Design review of the part built by this model. Coordinates are the model's own, in mm. Face numbers are marked on the shaded views. Give positions to 0.01 mm unless a question says otherwise; leave off trailing zeros. Loops run counter-clockwise (first coordinate to the right, second up) from the corner with the lowest first, then second, coordinate; pieces in that order, holes last. Notation, with made-up numbers: (85, 56.25) - (118, 56.25) arc R22 ccw to (118, 93.25) - close; hole circle Ø2 at (-9.75, -33.5). An arc over 180 degrees is marked (long way). Write each question's results on one line, items separated by ' | '.
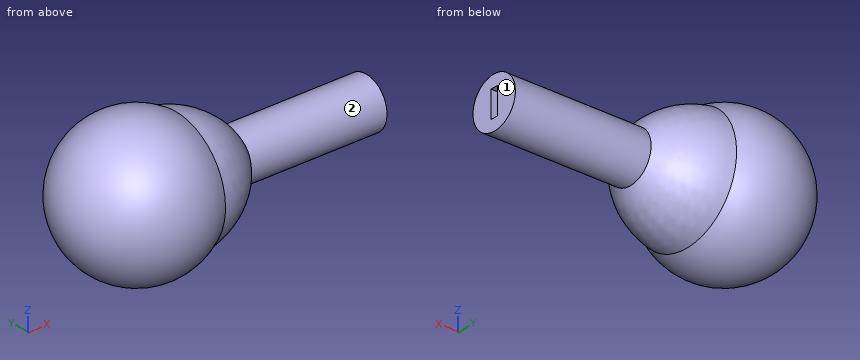
from build123d import *

# Parameters (mm, degrees)
SKETCH_2_W          = 5.3
SKETCH_2_H          = 1.5
CUT_EXTRUDE_2_DEPTH = 12


with BuildPart() as part:
    # 草图1 → 旋转4 (revolve)
    with BuildSketch(Plane.XY, mode=Mode.PRIVATE) as revolve_4_sk:
        with BuildLine():
            Line((-2.448374643, 5), (25, 5))
            Line((25, 5), (25, 0))
            Line((25, 0), (-35.778219949, 0))
            ThreePointArc((-35.778219949, 0), (-28.317806715, 12.571478645), (-13.708775535, 12.046075068))
            ThreePointArc((-13.708775535, 12.046075068), (-7.374475352, 9.64826615), (-2.448374643, 5))
        make_face()
    revolve(revolve_4_sk.sketch.rotate(Axis((-28.187562351, 0, 0), (1, 0, 0)), 90), axis=Axis((-28.187562351, 0, 0), (1, 0, 0)))

    # 草图2 → 切除-拉伸2 (cut)
    with BuildSketch(Plane(origin=(25, 0, 0), x_dir=(0, 0, -1), z_dir=(1, 0, 0))):
        Rectangle(SKETCH_2_W, SKETCH_2_H)
    extrude(amount=-CUT_EXTRUDE_2_DEPTH, mode=Mode.SUBTRACT)


solid = part.part
(1) Insertion check: P1, Ø12, axis at x = 0, z = -6.5, coming from the +Y side; P2, Ø1.2, axis at y = 0, z = 0.5, coming from the +X side; P3, Ø0.8, axis at x = 20.5, y = 0.5, coming from the -Z side. Each pin has a flat end and moves straight along its axis. Give the tip position at first contact, or say it passes through.
Answers below:
P1: y = 7.24 | P2: x = 13 | P3: z = -5
(2) Take a section at A-A on x = 12. Give the boundary of the cut face in (y, z).
Answers below:
outline: circle Ø10 at (0, 0)
(3) Take a section at B-B on x = -18.5. Give the boundary of the cut face in (y, z).
Answers below:
outline: circle Ø28.03 at (0, 0)
(4) Draft analysis for pull direction Y (two halves, no side actions). For the marked faces 1 and 2, state which applies: pulls with the +Y half, pulls with the -Y half, needs draft (parallel to the pull), parting line crosses it, or undercut.
Answers below:
face 1: needs draft | face 2: parting line crosses it
(5) Wall thickness on line 1 along Z through (x, y) = (-21, 7.75); line 2 along Y through (x, z) = (-6, 1.5); line 3 along X through (y, z) = (4.25, 12.5): over which ranges is each line inside the solid? List them lowest first. Write a range as from..to.
Answers below:
line 1: -12.04..12.04 | line 2: -8.56..8.56 | line 3: -27.01..-15.9
